```python
from build123d import *

# Parameters (mm, degrees)
F0_W     = 93
F0_H     = 55
F0_R     = 1.75
F1_DEPTH = 3
F2_W     = 93
F2_H     = 3
F2_H_2   = 15
F3_DEPTH = 15
F4_W     = 12
F4_H     = 12
F5_DEPTH = 15
F6_SIZE  = 2.5
F7_R     = 5


with BuildPart() as f1:
    # F0 (on Top) → F1 (new body)
    with BuildSketch(Plane.XY):
        with Locations((46.5, 27.5)):
            Rectangle(F0_W, F0_H)
        with Locations((18.325063, 34.906461)):
            Circle(F0_R, mode=Mode.SUBTRACT)
        with Locations((74.674937, 34.906461)):
            Circle(F0_R, mode=Mode.SUBTRACT)
    extrude(amount=F1_DEPTH)

    # F2 (on face) → F3 (join)
    with BuildSketch(Plane.XY.offset(3)):
        with Locations((46.5, 1.5)):
            Rectangle(F2_W, F2_H)
        with Locations((46.5, 47.5)):
            Rectangle(F2_W, F2_H_2)
    extrude(amount=F3_DEPTH)

    # F4 (on face) → F5 (cut, through all)
    with BuildSketch(Plane(origin=(0, 55, 0), x_dir=(-1, 0, 0), z_dir=(0, 1, 0))):
        with Locations((-84, 9)):
            Rectangle(F4_W, F4_H)
        with Locations((-69, 9)):
            Rectangle(F4_W, F4_H)
        with Locations((-54, 9)):
            Rectangle(F4_W, F4_H)
        with Locations((-39, 9)):
            Rectangle(F4_W, F4_H)
        with Locations((-24, 9)):
            Rectangle(F4_W, F4_H)
        with Locations((-9, 9)):
            Rectangle(F4_W, F4_H)
    extrude(amount=-F5_DEPTH, mode=Mode.SUBTRACT)

    # F6
    f6_edges = [f1.edges().sort_by_distance(p)[0] for p in [
        (16.575063, 34.906461, 3),
        (72.924937, 34.906461, 3),
    ]]
    chamfer(f6_edges, length=F6_SIZE)

    # F7
    f7_edges = [f1.edges().sort_by_distance(p)[0] for p in [
        (0, 47.5, 18),
        (93, 47.5, 18),
        (93, 1.5, 18),
        (0, 1.5, 18),
    ]]
    fillet(f7_edges, radius=F7_R)


solid = f1.part
```
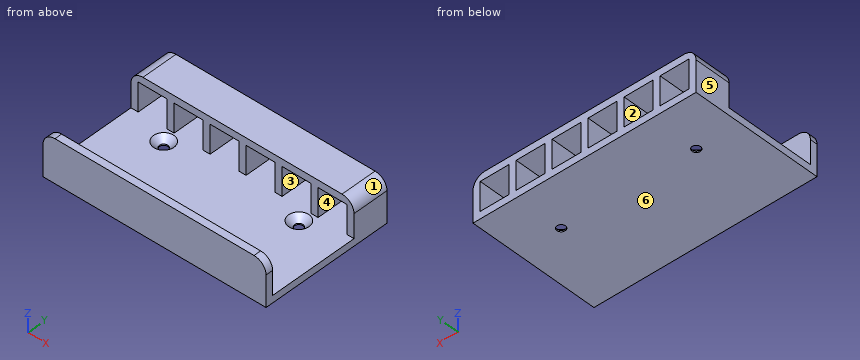
Work out the finished part from the listing and answer in its coordinate system (mm). Face numbers are marked on the shaded views. A direction names the side the tool comes from. Give positions to 0.01 mm unless a question says otherwise; leave off trailing zeros. Order: outer loops, then holes, each group sorted by start corner. A loop starts at its lowest first (then second) coordinate and runs counter-clockwise, first axis right, second up. Notation, with made-up numbers: M 23,61.25 L 52,61.25 A18 ccw 52,90.25 Z; hole C 23.25,78 d9. An arc over 180 degrees is marked long. Return JSON: item names as keys, results as strings.
1) For a pull along Z with two mould halves and no side action, classify the marked faces 3, 4, 5 and 6 as +Z half, -Z half, draft (parallel to the pull), parting line (faces both ways), or undercut.
Resolved:
{"face 3": "undercut", "face 4": "undercut", "face 5": "draft", "face 6": "-Z half"}
2) Straight lines are drawn through the part: line 1 along Y through (x, z) = (9.5, 15.25); line 2 along Z through (x, y) = (38, 45); line 3 along Z through (x, y) = (11, 18). For each, find the intervals that lie inside material, in ascending order. Write a range as [from, to].
Resolved:
{"line 1": "[0, 3], [40, 55]", "line 2": "[0, 3], [15, 18]", "line 3": "[0, 3]"}
3) Section B-B, the plane x = 54.5 is taken. Write down the section's boundary in (y, z), plus the area to 3 significant figures.
Resolved:
{"outline": "M 0,0 L 55,0 L 55,3 L 3,3 L 3,18 L 0,18 Z; M 40,15 L 55,15 L 55,18 L 40,18 Z", "area": "255 mm^2"}
4) Each of these flat-tipped pins is pushed along its axis until it touches: pin 1 (3 mm diameter, centred on x = 32.5, y = 20.5, fed in from +Z); pin 2 (2 mm diameter, centred on x = 83, z = 8, fed in from +Y). Where does it stop, or does it pass through?
Resolved:
{"pin 1": "z = 3", "pin 2": "y = 3"}
5) A tool of negligible diameter and unlimited length cuts with its end or side. For the marked faces 1 and 2, from which of +Z, -Z, +X, -X, +Y, -Y can it reach the whole face along a straight path? Write none if from no direction.
Resolved:
{"face 1": "+Z, +X, +Y, -Y", "face 2": "+Y"}
6) Section A-A, the plane z = 8.5 is taken. Give the number of separate pieces and of enclosed holes in the cut face, plus the area to 3 significant figures.
Resolved:
{"separate pieces": "8", "enclosed holes": "0", "area": "594 mm^2"}
7) Section D-D, the plane y = 17 is taken. Write down the section's boundary in (x, z).
Resolved:
{"outline": "M 0,0 L 93,0 L 93,3 L 0,3 Z"}
